Check sheet for the drawn part. Datum: minimum x, y, z corner. Units: mm. Coordinates: 2 decimals unless noted, no trailing zeros. Write each loop counter-clockwise with the first axis right and the second up, starting at its lowest first coordinate (ties: lowest second). Pieces come first, ordered by that corner, then holes. Notation, with made-up numbers: M 67.5,84 L 123.5,84 A34 cw 123.5,114 Z; hole C 22.25,79.5 d7. An arc over 180 degrees is marked long. Answer as CSV lines item,"result".
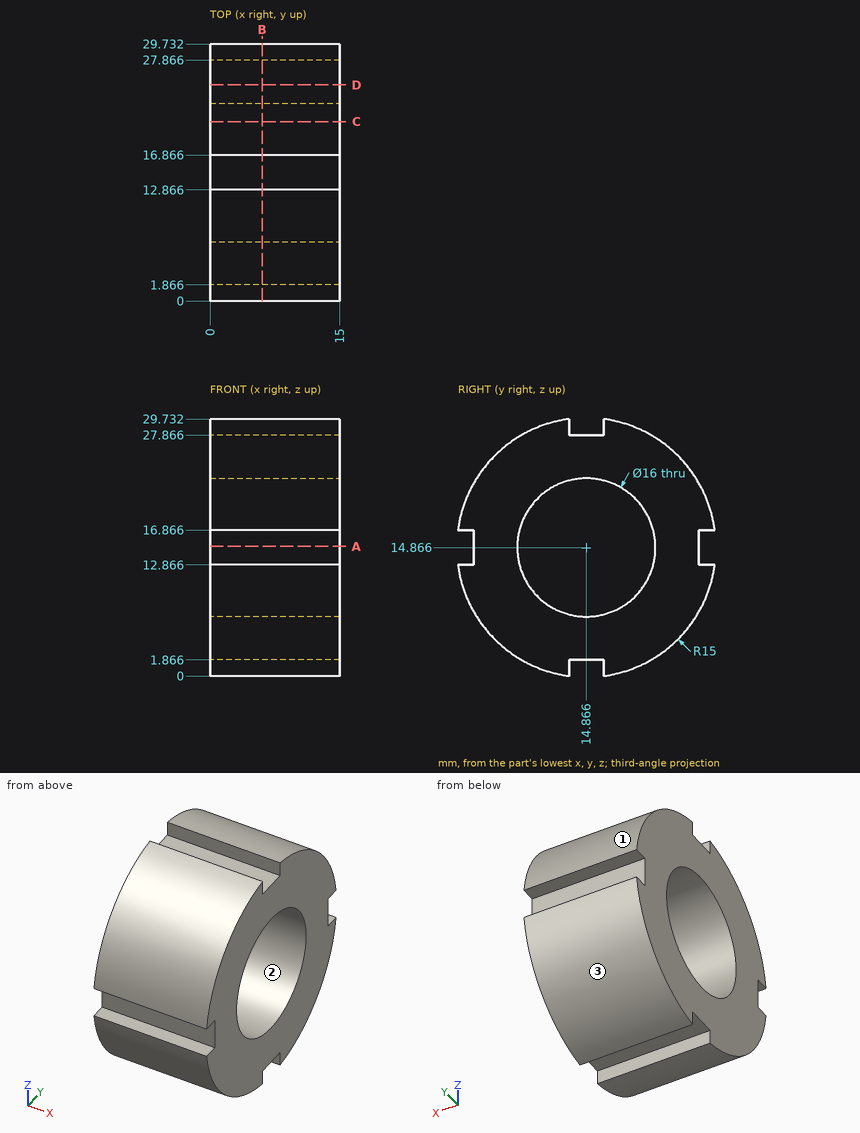
1) Thickness scan on line 1 along Y through (x, z) = (9, 9.25) (1 decimal); line 2 along Z through (x, y) = (5.75, 16.5) (1 decimal); line 3 along Y through (x, z) = (10, 15.25) (1 decimal). Record the ranges inside material, lowest first.
Answer key:
line 1,"y = 1 to 9.2, 20.6 to 28.8"
line 2,"z = 1.9 to 7, 22.7 to 27.9"
line 3,"y = 1.9 to 6.9, 22.9 to 27.9"
2) Section check D-D, the plane y = 25. Record the boundary of the cut face in (x, z) (3 decimals), plus the area to 3 significant figures.
Answer key:
outline,"M 0,3.807 L 15,3.807 L 15,25.925 L 0,25.925 Z"
area,"332 mm2"
3) Section check C-C, the plane y = 20.75. Record the boundary of the cut face in (x, z).
Answer key:
outline,"M 0,1.07 L 15,1.07 L 15,9.45 L 0,9.45 Z; M 0,20.29 L 15,20.29 L 15,28.66 L 0,28.66 Z"
4) Mould release check, pull along Z, two halves, no side actions. Record for the marked faces 1, 2 and 3: pulls with the +Z half, pulls with the -Z half, needs draft (parallel to the pull), parting line crosses it, or undercut.
Answer key:
face 1,"pulls with the +Z half"
face 2,"undercut"
face 3,"pulls with the -Z half"
5) Section check B-B, the plane x = 6. Record the boundary of the cut face in (y, z).
Answer key:
outline,"M 0,12.87 A15 ccw 12.87,0 L 12.87,1.87 L 16.87,1.87 L 16.87,0 A15 ccw 29.73,12.87 L 27.87,12.87 L 27.87,16.87 L 29.73,16.87 A15 ccw 16.87,29.73 L 16.87,27.87 L 12.87,27.87 L 12.87,29.73 A15 ccw 0,16.87 L 1.87,16.87 L 1.87,12.87 Z; hole C 14.87,14.87 d16"
6) Depth check by flat-ended pin: P1, Ø8, axis at y = 10.5, z = 12, coming from the -X side; P2, Ø3, axis at x = 5.5, y = 15, coming from the +Z side; P3, Ø6, axis at x = 6.5, z = 17, coming from the +Y side; P4, Ø0.6, axis at x = 4, z = 29, coming from the +Y side (1 decimal). Enter the tip coordinate at first touch or a pass-through.
Answer key:
P1,"stops at x = 0"
P2,"stops at z = 27.87"
P3,"stops at y = 29.73"
P4,"stops at y = 20.7"
7) Section check A-A, the plane z = 15. Record the boundary of the cut face in (x, y) (3 decimals).
Answer key:
outline,"M 0,1.866 L 15,1.866 L 15,6.867 L 0,6.867 Z; M 0,22.865 L 15,22.865 L 15,27.866 L 0,27.866 Z"
